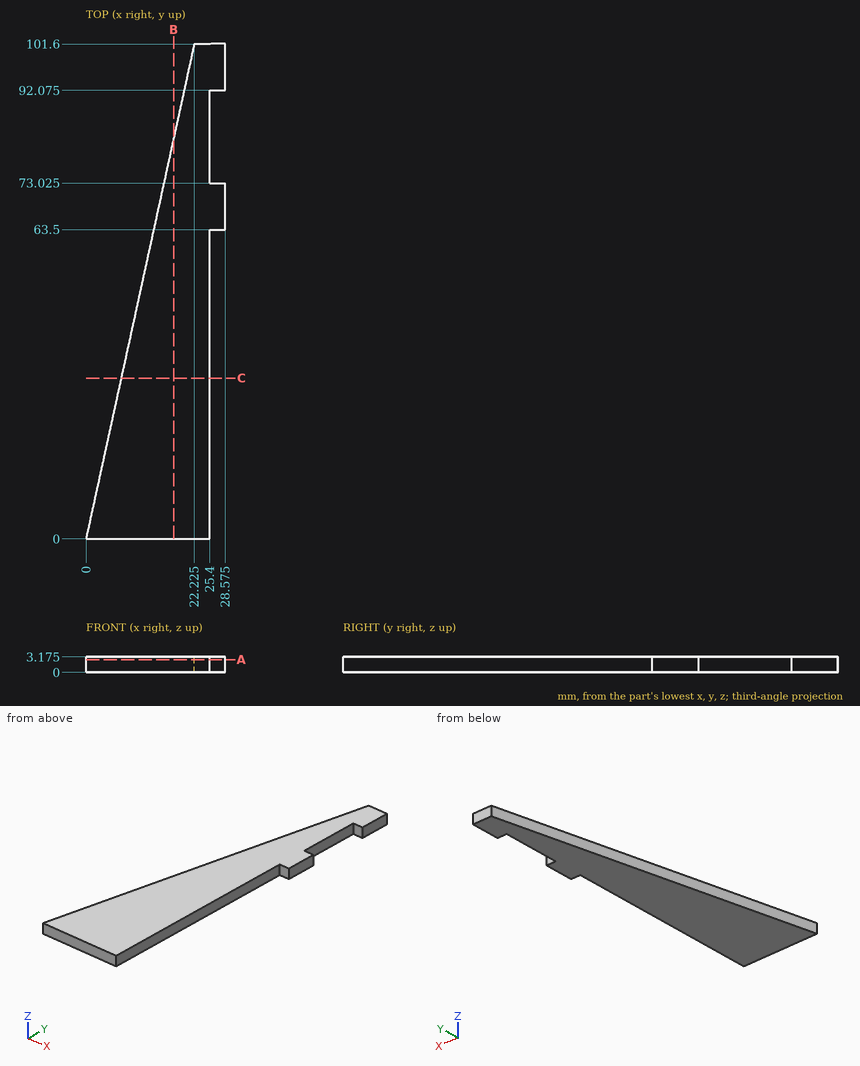
Verification items for this drawing (mm, ordinates from the low corner). Give positions to 0.01 mm unless a question says otherwise; leave off trailing zeros. Write each loop counter-clockwise with the first axis right and the second up, starting at its lowest first coordinate (ties: lowest second). Pieces come first, ordered by that corner, then holes. Notation, with made-up numbers: (74.5, 73) -> (120.5, 73) arc R20 cw to (120.5, 93) -> close; hole circle Ø4 at (2, 52). An arc over 180 degrees is marked (long way). Use CSV: the item, a comma, the result in double quotes.
(1) Sectioned sample at A-A (z = 2.6). Record the cut outline in (x, y) (3 decimals).
Derived:
outline,"(0, 0) -> (25.4, 0) -> (25.4, 63.5) -> (28.575, 63.5) -> (28.575, 73.025) -> (25.4, 73.025) -> (25.4, 92.075) -> (28.575, 92.075) -> (28.575, 101.6) -> (22.225, 101.6) -> close"
(2) Material ranges on L1, parallel to X at y = 9.5, z = 2.45; L2, parallel to X at y = 79.5, z = 0.5, recorded low to high.
Derived:
L1,"x = 2.08 to 25.4"
L2,"x = 17.39 to 25.4"
(3) Go/stop test with a flat-tipped pin: pin 1 (1.6 mm diameter, centred on y = 80, z = 1.5, fed in from +X). Record where the tip stops, or that it passes through.
Derived:
pin 1,"stops at x = 25.4"
(4) Sectioned sample at B-B (x = 18). Record the cut outline in (y, z) (3 decimals), plus the area to 3 significant figures.
Derived:
outline,"(0, 0) -> (82.286, 0) -> (82.286, 3.175) -> (0, 3.175) -> close"
area,"261 mm^2"
(5) Sectioned sample at C-C (y = 33). Record the cut outline in (x, z) (3 decimals).
Derived:
outline,"(7.219, 0) -> (25.4, 0) -> (25.4, 3.175) -> (7.219, 3.175) -> close"
